For this review, take the finished solid that the model builds, in its own axes (mm). Face numbers are marked on the shaded views. A direction names the side the tool comes from. Round coordinates to 2 decimals unless told otherwise and drop trailing zeros. Loops run counter-clockwise (first coordinate to the right, second up) from the corner with the lowest first, then second, coordinate; pieces in that order, holes last.
```python
from build123d import *

# Parameters (mm, degrees)
CROQUIS1_W              = 140
CROQUIS1_H              = 140
SALIENTE_EXTRUIR1_DEPTH = 40
CROQUIS3_W              = 130
CROQUIS3_H              = 130
CORTAR_EXTRUIR1_DEPTH   = 35
CROQUIS5_R              = 1.2
CROQUIS5_R_2            = 1.9
SALIENTE_EXTRUIR4_DEPTH = 50
CROQUIS6_W              = 5
CROQUIS6_H              = 5
CROQUIS6_W_2            = 4
CROQUIS6_H_2            = 4
SALIENTE_EXTRUIR5_DEPTH = 2


with BuildPart() as part:
    # Croquis1 → Saliente-Extruir1 (new body)
    with BuildSketch(Plane(origin=(0, 0, 0), x_dir=(1, 0, 0), z_dir=(0, 1, 0))):
        Rectangle(CROQUIS1_W, CROQUIS1_H)
    extrude(amount=SALIENTE_EXTRUIR1_DEPTH)

    # Croquis3 → Cortar-Extruir1 (cut)
    with BuildSketch(Plane(origin=(0, 40, 0), x_dir=(1, 0, 0), z_dir=(0, 1, 0))):
        Rectangle(CROQUIS3_W, CROQUIS3_H)
    extrude(amount=-CORTAR_EXTRUIR1_DEPTH, mode=Mode.SUBTRACT)

    # Croquis5 → Saliente-Extruir4 (add)
    with BuildSketch(Plane.XZ):
        with Locations(Location((-16, -64, 0), (0, 0, 90))):
            Circle(CROQUIS5_R)
        with Locations(Location((-16, 64, 0), (0, 0, 90))):
            Circle(CROQUIS5_R_2)
        with Locations(Location((20, 64, 0), (0, 0, 90))):
            Circle(CROQUIS5_R_2)
        with Locations(Location((20, -64, 0), (0, 0, 90))):
            Circle(CROQUIS5_R)
    extrude(amount=SALIENTE_EXTRUIR4_DEPTH)

    # Croquis6 → Saliente-Extruir5 (add)
    with BuildSketch(Plane.XZ.offset(50)):
        with Locations((-16, 64)):
            Rectangle(CROQUIS6_W, CROQUIS6_H)
        with Locations((20, 64)):
            Rectangle(CROQUIS6_W, CROQUIS6_H)
        with Locations((-16, -64)):
            Rectangle(CROQUIS6_W_2, CROQUIS6_H_2)
        with Locations((20, -64)):
            Rectangle(CROQUIS6_W_2, CROQUIS6_H_2)
    extrude(amount=SALIENTE_EXTRUIR5_DEPTH)


solid = part.part
```
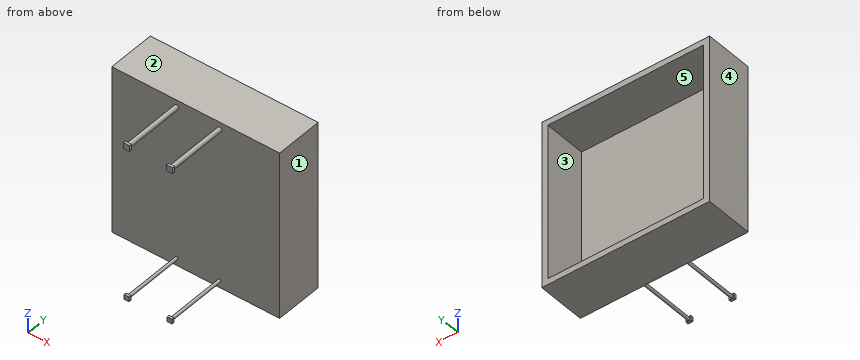
(1) For L1, parallel to Z at x = -15.5, y = 35; L2, parallel to Y at x = 12.5, z = 46.5, list the stretches that pass through material, from the lowest coordinate up.
(2) Add section B-B (z = 56). Give the boundary of the cut face in (x, y).
(3) For the marked faces 4 and 5, list the 3-axis set-ups (+Z, -Z, +X, -X, +Y, -Y) from which the entire face can be reached by the end or side of a thin tool; tool diameter is ignored.
(4) Add section A-A (y = 34). Give the boundary of the cut face in (x, z), plus the area to 3 significant figures.
(5) Add section C-C (x = 0). Give the boundary of the cut face in (y, z), plus the area to 3 significant figures.
(6) The part is to be moulded in two halves that separate along Z. For the marked faces 1, 2 and 3, say which applies: pulls with the +Z half, pulls with the -Z half, needs draft (parallel to the pull), parting line crosses it, or undercut.
(7) Insertion check: pin 1 Ø2 at (x, y) = (19, -50.5) entering from +Z; pin 2 Ø2 at (y, z) = (-51, -63.5) entering from +X; pin 3 Ø0.6 at (x, y) = (21, -50.5) entering from -Z. Each pin has a flat end and moves straight along its axis. Give the tip position at first contact, or say it passes through.
(8) Add section D-D (y = -9.5). Give the boundary of the cut face in (x, z).
Outcome:
1. L1: z = -70 to -65, 65 to 70
1. L2: y = 0 to 5
2. outline: (-70, 0) - (70, 0) - (70, 40) - (65, 40) - (65, 5) - (-65, 5) - (-65, 40) - (-70, 40) - close
3. face 4: +Z, -Z, -X, +Y, -Y
3. face 5: +Y
4. outline: (-70, -70) - (70, -70) - (70, 70) - (-70, 70) - close; hole (-65, -65) - (65, -65) - (65, 65) - (-65, 65) - close
4. area: 2,700 mm2
5. outline: (0, -70) - (40, -70) - (40, -65) - (5, -65) - (5, 65) - (40, 65) - (40, 70) - (0, 70) - close
5. area: 1,050 mm2
6. face 1: needs draft
6. face 2: pulls with the +Z half
6. face 3: undercut
7. pin 1: stops at z = 66.5
7. pin 2: stops at x = 22
7. pin 3: stops at z = -66
8. outline: circle Ø3.8 at (-16, 64); circle Ø2.4 at (-16, -64); circle Ø3.8 at (20, 64); circle Ø2.4 at (20, -64)
